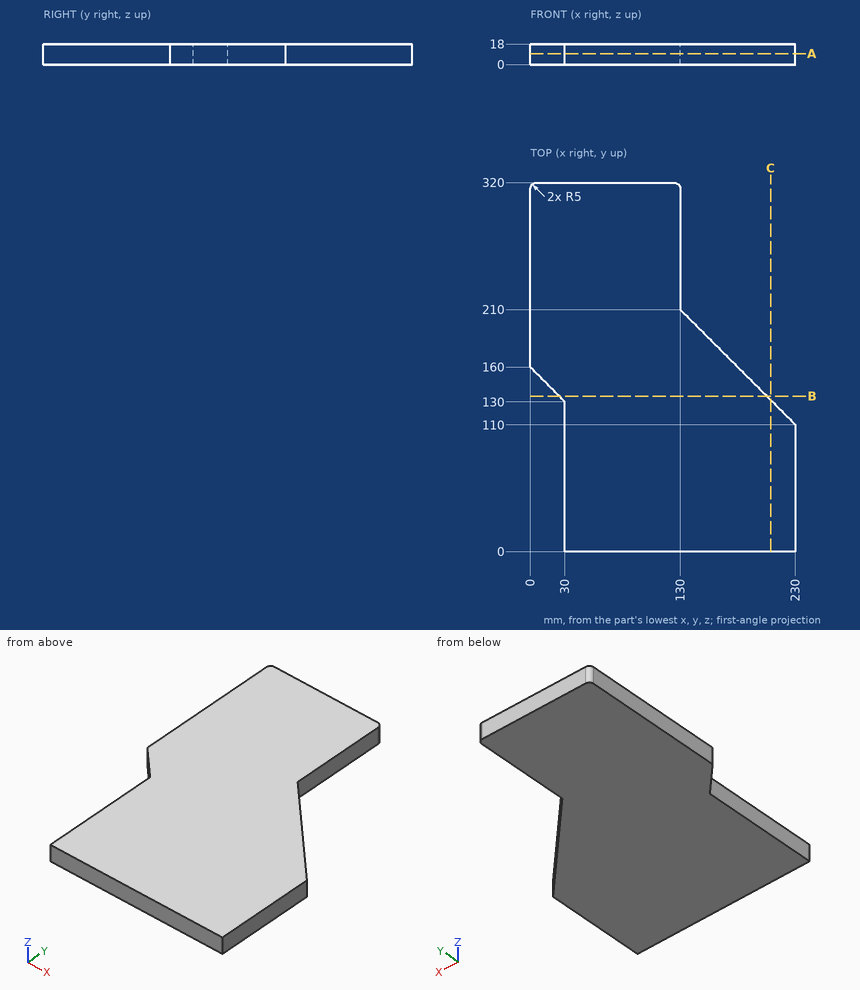
Input: dimensioned drawing with shaded views. Units: mm. Origin: part minimum x, y, z. Coordinates: 2 decimals unless noted, no trailing zeros. Order: outer loops, then holes, each group sorted by start corner. A loop starts at its lowest first (then second) coordinate and runs counter-clockwise, first axis right, second up. Notation, with made-up numbers: (13, 23.25) -> (17, 23.25) arc R22 cw to (17, 48.25) -> close; hole circle Ø4 at (11.25, 28.5). An arc over 180 degrees is marked (long way). Use CSV: the item, a comma, the result in double quotes.
1) Line query: line 1 (X direction, y = 214.5, z = 11.5); line 2 (X direction, y = 31, z = 13); line 3 (Y direction, x = 162, z = 6.5). Output: solid intervals per line, ascending.
Findings:
line 1,"x = 0 to 130"
line 2,"x = 30 to 230"
line 3,"y = 0 to 178"
2) Section B-B on y = 135. Output: boundary loops of the cut face in (x, z), then the cut area to 3 significant figures.
Findings:
outline,"(25, 0) -> (205, 0) -> (205, 18) -> (25, 18) -> close"
area,"3,240 mm^2"
3) Section C-C on x = 208.5. Output: boundary loops of the cut face in (y, z), then the cut area to 3 significant figures.
Findings:
outline,"(0, 0) -> (131.5, 0) -> (131.5, 18) -> (0, 18) -> close"
area,"2,370 mm^2"
4) Pin query (flat end, axial travel): pin 1 Ø2 at (x, z) = (130.5, 9.5) entering from +Y; pin 2 Ø6 at (y, z) = (235.5, 4.5) entering from +X; pin 3 Ø2 at (x, z) = (144, 4.5) entering from +Y. Return the tip coordinate at first contact, or that it passes through.
Findings:
pin 1,"stops at y = 317.18"
pin 2,"stops at x = 130"
pin 3,"stops at y = 197"
5) Section A-A on z = 9.75. Output: boundary loops of the cut face in (x, y).
Findings:
outline,"(0, 160) -> (30, 130) -> (30, 0) -> (230, 0) -> (230, 110) -> (130, 210) -> (130, 315) arc R5 ccw to (125, 320) -> (5, 320) arc R5 ccw to (0, 315) -> close"
